Solid Edge part; units mm, degrees
sketch "Sketch1" plane through (0, 0, 0) normal (0, -1, 0) x (1, 0, 0)
  circle A0 centre (0, 0) radius 2
  circle A1 centre (0, 9.02) radius 2
  line L0 (3.5, -4) -> (3.5, 96)
  line L1 (3.5, 96) -> (-3.5, 96)
  line L2 (-3.5, 96) -> (-3.5, -4)
  line L3 (-3.5, -4) -> (3.5, -4)
extrude "Protrusion1" add sketch "Sketch1" against normal blind 7
sketch "Sketch2" plane through (3.5, 3.5, 46) normal (1, 0, 0) x (0, 0, -1)
  line L0 (-30, 3.5) -> (-26.4645, -0.0355)
  line L1 (-26.4645, -0.0355) -> (-22.9289, 3.5)
  line L2 (-22.9289, 3.5) -> (-30, 3.5)
extrude "ExtrudedCutout_1" cut sketch "Sketch2" against normal blind 24
sketch "Sketch3" plane through (3.5, 3.5, 46) normal (1, 0, 0) x (0, 0, -1)
  line L0 (-31.4645, -3.5) -> (-21.4645, -3.5)
  arc A0 (-21.4645, -3.5) -> (-31.4645, -3.5) centre (-26.4645, -3.5) cw
extrude "ExtrudedProtrusion_2" add sketch "Sketch3" against normal blind 7
fillet "Round_1" radius 3 2 edges at (0, 0, 67.4645) (0, 0, 77.4645)
fillet "Round_2" radius 1 4 edges at (0, 7, 96) (0, 0, 96) (0, 0, -4) (0, 7, -4)
Model file for the job. Use its own axes, mm. A direction names the side the tool comes from. Coordinates: 2 decimals unless noted, no trailing zeros. Loops run counter-clockwise (first coordinate to the right, second up) from the corner with the lowest first, then second, coordinate; pieces in that order, holes last. Notation, with made-up numbers: (43.5, -2) -> (79.5, -2) arc R18 ccw to (79.5, 25) -> close; hole circle Ø8 at (-2, -27). An arc over 180 degrees is marked (long way). Use one line per item in the form item = value. Start each with the question number.
(1) Tool access for faces 1 (the flat face through (0, 0, 32)), 2 (the flat face through (0, 0, 88)), 3 (the flat face through (0.05, 5.21, 70.72)): list every direction of +Z, -Z, +X, -X, +Y, -Y with a clear straight run to the whole face (end or side of a thin tool).
(2) Pull direction X, two halves, no side cores. Call faces 4 (the flat face through (0, 7, 86)), 5 (the flat face through (-3.5, 4, 47)), 6 (the cylindrical face through (0, 3, -2)): pulls with the +X half, pulls with the -X half, needs draft (parallel to the pull), parting line crosses it, or undercut.
(3) Cut at D-D on z = 61. Give the cut face in (x, y).
(4) Cut at B-B on z = 0. Give the cut face in (x, y), and give its area (3 significant figures).
(5) Flat gauge pins, fed straight in: pin 1 (1.5 mm diameter, centred on x = 1.5, z = 18.5, fed in from -Y); pin 2 (3.5 mm diameter, centred on x = 0, z = 9.02, fed in from +Y); pin 3 (4 mm diameter, centred on x = 0.5, y = -1, fed in from -Z). Where does each tip first touch, or does it go through?
(6) Cut at A-A on x = 0. Give the cut face in (y, z) (1 decimal).
(7) Cut at C-C on y = 2.25. Give the cut face in (x, z), and give its area (3 significant figures).
(8) Probe probe 1 along Z at (x, y) = (0, 2.75); probe 2 along Z at (x, y) = (0, 4.5); probe 3 along Z at (x, y) = (0, 4.25). List the from-to ranges inside material, lowest first. Write a range as from..to.
Values:
q1.face_1 = -Z, +X, -X, -Y
q1.face_2 = +Z, +X, -X, -Y
q1.face_3 = +X, -X, +Y
q2.face_4 = needs draft
q2.face_5 = pulls with the -X half
q2.face_6 = undercut
q3.outline = (-3.5, 0) -> (3.5, 0) -> (3.5, 7) -> (-3.5, 7) -> close
q4.outline = (-3.5, 0) -> (-2, 0) -> (-2, 7) -> (-3.5, 7) -> close; (2, 0) -> (3.5, 0) -> (3.5, 7) -> (2, 7) -> close
q4.area = 21.0 mm2
q5.pin_1 = 0
q5.pin_2 = through
q5.pin_3 = -4
q6.outline = (-1.9, 67.8) arc R3 cw to (0, 65) -> (0, 11) -> (7, 11) -> (7, 68.9) -> (3.5, 72.5) -> (7, 76) -> (7, 95) arc R1 ccw to (6, 96) -> (1, 96) arc R1 ccw to (0, 95) -> (0, 79.9) arc R3 cw to (-1.9, 77.1) arc R5 ccw to start; (0, -3) arc R1 ccw to (1, -4) -> (6, -4) arc R1 ccw to (7, -3) -> (7, -2) -> (0, -2) -> close; (0, 2) -> (7, 2) -> (7, 7) -> (0, 7) -> close
q7.outline = (-3.5, -4) -> (3.5, -4) -> (3.5, 96) -> (-3.5, 96) -> close; hole circle Ø4 at (0, 0); hole circle Ø4 at (0, 9.02)
q7.area = 675 mm2
q8.probe_1 = -4..-2, 2..7.02, 11.02..96
q8.probe_2 = -4..-2, 2..7.02, 11.02..71.43, 73.5..96
q8.probe_3 = -4..-2, 2..7.02, 11.02..71.68, 73.25..96
